Source: CAD feature listing. Evaluate the final solid. Frame: model axes, mm. A direction names the side the tool comes from. Coordinates: 2 decimals unless noted, no trailing zeros. Loops run counter-clockwise (first coordinate to the right, second up) from the corner with the lowest first, then second, coordinate; pieces in that order, holes last. Notation, with made-up numbers: (32, 18) -> (64, 18) arc R28 ccw to (64, 41) -> close; hole circle Ø10 at (50, 85). An arc over 180 degrees is marked (long way). Answer as CSV lines item,"result".
from build123d import *

# Parameters (mm, degrees)
BOSS_EXTRUDE1_DEPTH = 25
CUT_EXTRUDE1_REACH  = 16
SKETCH2_R           = 7
BOSS_EXTRUDE2_DEPTH = 14


with BuildPart() as part:
    # Sketch1 → Boss-Extrude1 (new body, symmetric)
    with BuildSketch(Plane(origin=(0, 0, 0), x_dir=(0, 0, -1), z_dir=(1, 0, 0))):
        Polygon((0, 0), (0, 14), (28, 14), (28, 0), (21, 0), (21, 7), (7, 7), (7, 0), align=None)
    extrude(amount=BOSS_EXTRUDE1_DEPTH, both=True)

    # Sketch2 → Cut-Extrude1 (cut, up to next)
    with BuildSketch(Plane(origin=(0, 14, 0), x_dir=(1, 0, 0), z_dir=(0, 1, 0)), mode=Mode.PRIVATE) as cut_extrude1_sk1:
        with Locations((11, 14)):
            Circle(SKETCH2_R)
    cut_extrude1_tool1 = extrude(cut_extrude1_sk1.sketch, amount=-CUT_EXTRUDE1_REACH, mode=Mode.PRIVATE) & part.part
    add(cut_extrude1_tool1.solids().sort_by_distance((11, 14, -14))[0], mode=Mode.SUBTRACT)

    # Sketch3 → Boss-Extrude2 (add)
    with BuildSketch(Plane(origin=(0, 14, 0), x_dir=(1, 0, 0), z_dir=(0, 1, 0))):
        Polygon((-4, 14), (-4, 28), (-25, 28), (-25, 0), (-11, 0), (-11, 14), align=None)
    extrude(amount=BOSS_EXTRUDE2_DEPTH)


solid = part.part
(1) Cut plane D-D (z = -2). Return the cut outline in (x, y).
Computed values:
outline,"(-25, 0) -> (25, 0) -> (25, 14) -> (-11, 14) -> (-11, 28) -> (-25, 28) -> close"
(2) Material intervals for L1, parallel to X at y = 10.25, z = -14; L2, parallel to Z at x = 20, y = 2.5; L3, parallel to Y at x = -5, z = -9.5, sorted ascending. Write a range as [from, to].
Computed values:
L1,"[-25, 4], [18, 25]"
L2,"[-28, -21], [-7, 0]"
L3,"[7, 14]"
(3) Draft query along Z for faces 1 (the flat face through (0, 3, -21)), 2 (the flat face through (0, 0, -25)), 3 (the flat face through (-5, 11, -28)). Return one class per face: released by +Z, released by -Z, zero draft, split by the parting line, or undercut.
Computed values:
face 1,"undercut"
face 2,"zero draft"
face 3,"released by -Z"
(4) Cut plane C-C (x = -21). Return the cut outline in (y, z).
Computed values:
outline,"(0, -28) -> (28, -28) -> (28, 0) -> (0, 0) -> (0, -7) -> (7, -7) -> (7, -21) -> (0, -21) -> close"
(5) Access query for faces 4 (the flat face through (-17, 28, -14)), 5 (the flat face through (21, 7, -14)), 6 (the flat face through (-25, 14, -14)), 7 (the flat face through (-4, 21, -21)), 8 (the flat face through (-11, 21, -7)). Directions: +Z, -Z, +X, -X, +Y, -Y. A direction counts if a zero-diameter tool reaches every point of the face in a straight line with its end or side. Return the directions, or none.
Computed values:
face 4,"+Z, -Z, +X, -X, +Y"
face 5,"+X, -X, -Y"
face 6,"+Z, -Z, -X, +Y, -Y"
face 7,"+Z, -Z, +X, +Y"
face 8,"+Z, +X, +Y"
(6) Cut plane A-A (x = 9). Return the cut outline in (y, z), then the cut area to 3 significant figures.
Computed values:
outline,"(0, -28) -> (14, -28) -> (14, -20.71) -> (7, -20.71) -> (7, -21) -> (0, -21) -> close; (0, -7) -> (7, -7) -> (7, -7.29) -> (14, -7.29) -> (14, 0) -> (0, 0) -> close"
area,"200 mm^2"
(7) Pin query (flat end, axial travel): pin 1 Ø11 at (y, z) = (20, -21) entering from +X; pin 2 Ø7 at (x, z) = (-4.5, -15) entering from -Y; pin 3 Ø3.5 at (x, y) = (-6, 18.5) entering from +Z; pin 4 Ø1.5 at (x, y) = (18, 15.5) entering from +Z. Return the tip coordinate at first contact, or that it passes through.
Computed values:
pin 1,"x = -4"
pin 2,"y = 7"
pin 3,"z = -14"
pin 4,"through"
(8) Cut plane B-B (z = -12). Return the cut outline in (x, y), then the cut area to 3 significant figures.
Computed values:
outline,"(-25, 7) -> (4.29, 7) -> (4.29, 14) -> (-11, 14) -> (-11, 28) -> (-25, 28) -> close; (17.71, 7) -> (25, 7) -> (25, 14) -> (17.71, 14) -> close"
area,"452 mm^2"
